from build123d import *

# Parameters (mm, degrees)
SKETCH3_R               = 0.5
CUT_EXTRUDE2_DEPTH      = 1.25
CUT_EXTRUDE2_DEPTH_BACK = 5.25


with BuildPart() as part:
    # Sketch1 → Revolve1 (revolve)
    with BuildSketch(Plane(origin=(0, 0, 0), x_dir=(1, 0, 0), z_dir=(0, 1, 0))):
        Polygon((0, 0), (4.5, 0), (4.5, 0.5), (5, 0.5), (5, 1.25), (3.25, 1.75), (1.25, 1.75), (-0.5, 1.25), (-0.5, 0.5), (0, 0.5), align=None)
    revolve(axis=Axis((0, 0, 0.5), (1, 0, 0)))

    # Sketch3 → Cut-Extrude2 (cut, two sides)
    with BuildSketch(Plane(origin=(0, 2, 0), x_dir=(1, 0, 0), z_dir=(0, 1, 0))) as cut_extrude2_sk:
        with Locations((2.25, -0.5)):
            Circle(SKETCH3_R)
    extrude(amount=CUT_EXTRUDE2_DEPTH, mode=Mode.SUBTRACT)
    extrude(cut_extrude2_sk.sketch, amount=-CUT_EXTRUDE2_DEPTH_BACK, mode=Mode.SUBTRACT)


solid = part.part
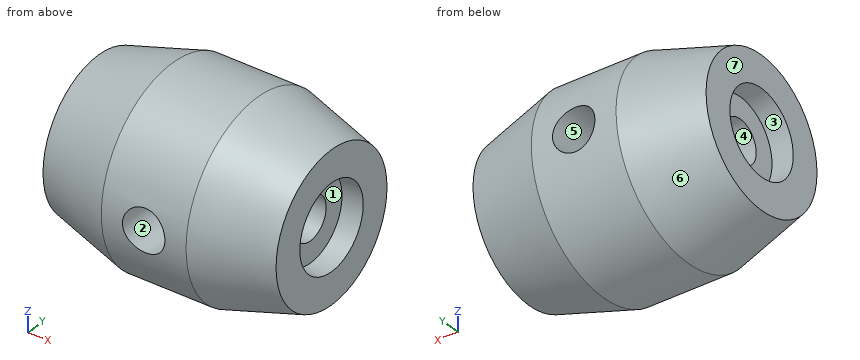
Input: part model. Units: mm. Frame: model coordinates. Face numbers are marked on the shaded views. A direction names the side the tool comes from. Round coordinates to 2 decimals unless told otherwise and drop trailing zeros. Loops run counter-clockwise (first coordinate to the right, second up) from the corner with the lowest first, then second, coordinate; pieces in that order, holes last. Notation, with made-up numbers: (21, 20) -> (51, 20) arc R14 ccw to (51, 27) -> close; hole circle Ø4 at (43.5, 49.5). An arc over 180 degrees is marked (long way). Answer as a JSON object with one key per item and string values. Group by question number.
1) Ray query, L1, parallel to X at y = -1.5, z = 0.5; L2, parallel to Y at x = 4.95, z = 0.5; L3, parallel to Z at x = 2.25, y = 0.7. Return the intervals inside material, ascending.
2) Section query B-B on x = 0.5. Output: boundary loops of the cut face in (y, z).
3) Section query C-C on x = 3.9. Output: boundary loops of the cut face in (y, z).
4) Draft query along Z for the marked faces 4, 5, 6 and 7. Return one class per face: +Z half, -Z half, draft (parallel to the pull), parting line (faces both ways), or undercut.
5) Reachability of the marked faces 1, 2 and 3 from +Z, -Z, +X, -X, +Y, -Y: full face, straight path, thin tool, end or side. Return the list, or none.
6) Pin query (flat end, axial travel): pin 1 (1.5 mm diameter, centred on x = 4, z = 0, fed in from -Y); pin 2 (2 mm diameter, centred on x = 3.5, y = -1.5, fed in from +Z). Return the tip coordinate at first contact, or that it passes through.
7) Section query A-A on z = 0.5. Output: boundary loops of the cut face in (x, y).
Reply:
{
 "1": {"L1": "x = -0.5 to 1.75, 2.75 to 5", "L2": "y = -1.76 to -1, 1 to 1.76", "L3": "z = -1.64 to 0, 1 to 2.64"},
 "2": {"outline": "circle Ø4.07 at (0, 0.5); hole circle Ø1 at (0, 0.5)"},
 "3": {"outline": "circle Ø4.13 at (0, 0.5); hole circle Ø1 at (0, 0.5)"},
 "4": {"face 4": "undercut", "face 5": "undercut", "face 6": "parting line", "face 7": "draft"},
 "5": {"face 1": "+X", "face 2": "+Y, -Y", "face 3": "-X"},
 "6": {"pin 1": "stops at y = -2.22", "pin 2": "stops at z = 2.69"},
 "7": {"outline": "(-0.5, -1.75) -> (1.25, -2.25) -> (1.75, -2.25) -> (1.75, -0.5) -> (0, -0.5) -> (0, -1) -> (-0.5, -1) -> close; (-0.5, 1) -> (0, 1) -> (0, 0.5) -> (1.75, 0.5) -> (1.75, 2.25) -> (1.25, 2.25) -> (-0.5, 1.75) -> close; (2.75, -2.25) -> (3.25, -2.25) -> (5, -1.75) -> (5, -1) -> (4.5, -1) -> (4.5, -0.5) -> (2.75, -0.5) -> close; (2.75, 0.5) -> (4.5, 0.5) -> (4.5, 1) -> (5, 1) -> (5, 1.75) -> (3.25, 2.25) -> (2.75, 2.25) -> close"}
}
